Model file for the job. Use its own axes, mm. A direction names the side the tool comes from. Round coordinates to 2 decimals unless told otherwise and drop trailing zeros. Use a Markdown table: item, result. Add a question column.
Autodesk Inventor part; units mm, degrees
ref_plane "Start Plane" through (0, 0, 0) normal (0, 0, 1) x (1, 0, 0)
ref_plane "End Plane" through (0, 0, 275) normal (0, 0, 1) x (1, 0, 0)
ref_plane "YZ Plane" through (0, 0, 0) normal (1, 0, 0) x (0, 1, 0)
ref_plane "Start Plane" through (0, 0, 0) normal (0, 0, 1) x (1, 0, 0)
ref_plane "End Plane" through (0, 0, 275) normal (0, 0, 1) x (1, 0, 0)
sketch "Sketch" plane through (0, 0, 0) normal (0, 0, 1) x (1, 0, 0)
  line L0 (10, -4.5951) -> (10, -8.2)
  line L1 (-10, -8.2) -> (-10, -4.5951)
  line L2 (-10, 10) -> (10, -10) construction
  line L3 (10, 10) -> (-10, -10) construction
  circle A0 centre (0, 0) radius 2.1
  line L4 (-2.84, -3.9007) -> (2.84, -3.9007)
  line L5 (3.9007, -2.84) -> (3.9007, 2.84)
  line L6 (2.84, 3.9007) -> (-2.84, 3.9007)
  line L7 (-3.9007, 2.84) -> (-3.9007, -2.84)
  line L8 (-3.9007, -3.9007) -> (3.9007, 3.9007) construction
  line L9 (3.9007, -3.9007) -> (-3.9007, 3.9007) construction
  line L10 (-3.9007, -2.84) -> (-2.84, -3.9007) construction
  line L11 (-2.84, -3.9007) -> (-5.4993, -6.56)
  line L12 (-5.4993, -6.56) -> (-5.4993, -8.2)
  line L13 (-5.4993, -8.2) -> (-2.7951, -8.2)
  line L14 (-2.7951, -8.2) -> (-4.5951, -10)
  line L15 (0, 0) -> (0, -3.9007) construction
  line L16 (3.9007, -2.84) -> (2.84, -3.9007) construction
  line L17 (2.84, -3.9007) -> (5.4993, -6.56)
  line L18 (5.4993, -6.56) -> (5.4993, -8.2)
  line L19 (5.4993, -8.2) -> (2.7951, -8.2)
  line L20 (2.7951, -8.2) -> (4.5951, -10)
  line L21 (-2.84, -3.9007) -> (-3.9007, -2.84) construction
  line L22 (-3.9007, -2.84) -> (-6.56, -5.4993)
  line L23 (-6.56, -5.4993) -> (-8.2, -5.4993)
  line L24 (-8.2, -5.4993) -> (-8.2, -2.7951)
  line L25 (-8.2, -2.7951) -> (-10, -4.5951)
  line L26 (3.9007, -2.84) -> (6.56, -5.4993)
  line L27 (6.56, -5.4993) -> (8.2, -5.4993)
  line L28 (8.2, -5.4993) -> (8.2, -2.7951)
  line L29 (8.2, -2.7951) -> (10, -4.5951)
  arc A1 (-10, -8.2) -> (-8.2, -10) centre (-8.2, -8.2) ccw
  arc A2 (8.2, -10) -> (10, -8.2) centre (8.2, -8.2) ccw
  line L30 (-8.2, -6.56) -> (-7.7111, -6.56)
  line L31 (-6.6505, -8.2) -> (-8.2, -8.2)
  line L32 (-8.2, -8.2) -> (-8.2, -6.56)
  line L33 (-6.6505, -7.6207) -> (-7.7111, -6.56)
  line L34 (-6.6505, -7.6207) -> (-6.6505, -8.2)
  line L35 (8.2, -6.56) -> (7.7111, -6.56)
  line L36 (6.6505, -8.2) -> (8.2, -8.2)
  line L37 (8.2, -8.2) -> (8.2, -6.56)
  line L38 (6.6505, -7.6207) -> (7.7111, -6.56)
  line L39 (6.6505, -7.6207) -> (6.6505, -8.2)
  line L40 (8.2, -10) -> (4.5951, -10)
  line L41 (-4.5951, -10) -> (-8.2, -10)
  line L42 (-3.9007, 0) -> (3.9007, 0) construction
  line L43 (10, 4.5951) -> (10, 8.2)
  line L44 (-10, 8.2) -> (-10, 4.5951)
  line L45 (-2.84, 3.9007) -> (2.84, 3.9007)
  line L46 (-3.9007, 2.84) -> (-2.84, 3.9007) construction
  line L47 (-2.84, 3.9007) -> (-5.4993, 6.56)
  line L48 (-5.4993, 6.56) -> (-5.4993, 8.2)
  line L49 (-5.4993, 8.2) -> (-2.7951, 8.2)
  line L50 (-2.7951, 8.2) -> (-4.5951, 10)
  line L51 (2.84, 3.9007) -> (5.4993, 6.56)
  line L52 (5.4993, 6.56) -> (5.4993, 8.2)
  line L53 (5.4993, 8.2) -> (2.7951, 8.2)
  line L54 (2.7951, 8.2) -> (4.5951, 10)
  line L55 (3.9007, 2.84) -> (2.84, 3.9007) construction
  line L56 (-8.2, 2.7951) -> (-10, 4.5951)
  line L57 (-2.84, 3.9007) -> (-3.9007, 2.84) construction
  line L58 (-3.9007, 2.84) -> (-6.56, 5.4993)
  line L59 (-6.56, 5.4993) -> (-8.2, 5.4993)
  line L60 (-8.2, 5.4993) -> (-8.2, 2.7951)
  line L61 (3.9007, 2.84) -> (6.56, 5.4993)
  line L62 (6.56, 5.4993) -> (8.2, 5.4993)
  line L63 (8.2, 5.4993) -> (8.2, 2.7951)
  line L64 (8.2, 2.7951) -> (10, 4.5951)
  arc A3 (-8.2, 10) -> (-10, 8.2) centre (-8.2, 8.2) ccw
  arc A4 (10, 8.2) -> (8.2, 10) centre (8.2, 8.2) ccw
  line L65 (-8.2, 6.56) -> (-7.7111, 6.56)
  line L66 (-6.6505, 8.2) -> (-8.2, 8.2)
  line L67 (-8.2, 8.2) -> (-8.2, 6.56)
  line L68 (-6.6505, 7.6207) -> (-7.7111, 6.56)
  line L69 (-6.6505, 7.6207) -> (-6.6505, 8.2)
  line L70 (8.2, 6.56) -> (7.7111, 6.56)
  line L71 (6.6505, 7.6207) -> (7.7111, 6.56)
  line L72 (8.2, 8.2) -> (8.2, 6.56)
  line L73 (6.6505, 7.6207) -> (6.6505, 8.2)
  line L74 (6.6505, 8.2) -> (8.2, 8.2)
  line L75 (8.2, 10) -> (4.5951, 10)
  line L76 (-4.5951, 10) -> (-8.2, 10)
  line L77 (-8.2, 10) -> (-4.5951, 10)
  line L78 (4.5951, 10) -> (8.2, 10)
  point P0 (8.2, -8.2)
  point P1 (0, 3.9007)
  point P2 (8.2, 8.2)
  dimension "Width" = 20
  dimension "Height" = 20
  dimension "d2" = 4.2
  dimension "d3" = 1.5
  dimension "d4" = 1.64
  dimension "d6" = 5.68
  dimension "d7" = 1.8
  dimension "d9" = 1.5
extrude "Body" add sketch "Sketch" along normal up to surface (275 mm away) from surface at 0
sketch "Sketch4" plane through (0, 0, 0) normal (0, 0, 1) x (1, 0, 0)
  line L0 (0, 0) -> (10, 0)
ref_plane "Work Plane4" through (0, 0, 0) normal (0, -1, 0) x (1, 0, 0)
sketch "Sketch5" plane through (0, 0, 0) normal (0, -1, 0) x (1, 0, 0)
  line L0 (-2, 0) -> (12, 0) construction
  line L1 (-2, 275) -> (12, 275) construction
  dimension "d17" = 275
equation "\"G_OFFSET_START\" = 0"
equation "\"G_OFFSET_END\" = 0"
equation "\"d13\" = Length + G_OFFSET_END"
equation "\"G_L\" = d17"
properties part number "V-slot 20 mm x 20 mm" material "Aluminum 6061"
1) Cut at A-A on z = 224. Count the separate pieces of the cut face and the enclosed holes in it, and give its area (3 significant figures).
2) Tool access for faces 4 (the face through (0, 3.901, 136)), 5 (the face through (2.003, -0.631, 135.575)), 6 (the face through (3.901, 0, 136)): list every direction of +Z, -Z, +X, -X, +Y, -Y with a clear straight run to the whole face (end or side of a thin tool).
3) Pin check, flat tips, straight feed: pin 1 Ø0.8 at (x, z) = (-4.5, 88) entering from -Y; pin 2 Ø6 at (x, z) = (1, 165) entering from +Y; pin 3 Ø6 at (x, z) = (1.5, 194.5) entering from -Y. Stop position of each tip, or through.
4) Pull direction X, two halves, no side cores. Call faces 1 (the face through (0, -3.901, 136)), 2 (the face through (-3.901, 0, 136)), 3 (the face through (-0.1, 2.4, 0)): +X half, -X half, draft (parallel to the pull), parting line (faces both ways), or undercut.
5) Wall check: probe 1 along Y at (x, z) = (0, 92.5); probe 2 along X at (y, z) = (8.25, 122); probe 3 along X at (y, z) = (-5.25, 155.5). Give the ranges that are in metal, low to high. Write a range as from..to.
Established:
| question | item | result |
|---|---|---|
| 1 | separate pieces | 1 |
| 1 | enclosed holes | 5 |
| 1 | area | 161 mm^2 |
| 2 | face 4 | +Z, -Z, +Y |
| 2 | face 5 | +Z, -Z |
| 2 | face 6 | +Z, -Z, +X |
| 3 | pin 1 | stops at y = -10 |
| 3 | pin 2 | stops at y = 9.4 |
| 3 | pin 3 | stops at y = -9.9 |
| 4 | face 1 | undercut |
| 4 | face 2 | -X half |
| 4 | face 3 | draft |
| 5 | probe 1 | y = -3.9..-2.1, 2.1..3.9 |
| 5 | probe 2 | x = -10..-2.85, 2.85..10 |
| 5 | probe 3 | x = -10..-8.2, -6.31..-4.19, 4.19..6.31, 8.2..10 |
